Could you check a few things on this model? Use its own coordinates, in mm. A direction names the side the tool comes from. Round coordinates to 2 decimals unless told otherwise and drop trailing zeros. Write each loop counter-clockwise with the first axis right and the second up, starting at its lowest first coordinate (ties: lowest second). Pieces come first, ordered by that corner, then holes. Notation, with made-up numbers: M -17.75,-15 L 23.25,-15 A18 ccw 23.25,7 Z; hole C 22,48.5 d1. An arc over 180 degrees is marked long. One line per item, written item: value. Start each with the question number.
(1) Which directions (+Z, -Z, +X, -X, +Y, -Y) give clear straight access to the entire face, cutting with the end or side of a thin tool? Please do faces 4 (the face through (7, -66, 30)), 5 (the face through (1074.98, 1.66, 14.79)).
(2) Thinking about a two-plate mould opening in Y: for faces 1 (the face through (7, -66, 0)), 2 (the face through (1089.98, 1.99, 14.79)), 3 (the face through (-1049.99, -1.09, 14.79)), which applies, released by +Y, released by -Y, zero draft, split by the parting line, or undercut?
(3) I want a section at B-B on x = 436. Please give me the cut outline in (y, z).
(4) I want a section at C-C on z = 24. Please give me the cut outline in (x, y) (1 decimal), and give its area (3 significant figures).
(5) I want a section at A-A on y = 0. Please give me the cut outline in (x, z).
(6) I'm going to push flat-ended pins straight in: pin 1 Ø1 at (x, z) = (529, 23.5) entering from +Y; pin 2 Ø1.5 at (y, z) = (25, 26) entering from -X; pin 3 Ø4 at (y, z) = (44.5, 10.5) entering from -X. Where does each tip first touch, or does it pass through?
(7) If I drill on L1, parallel to X at y = 2.5, z = 17; L2, parallel to Y at x = 65.5, z = 23.75; L3, parallel to Y at x = -871, z = 24.5, over which ranges is the centre line in solid material (lowest first)?
Autodesk Inventor part; units mm, degrees
ref_plane "YZ Plane" through (0, 0, 0) normal (1, 0, 0) x (0, 1, 0)
ref_plane "XZ Plane" through (0, 0, 0) normal (0, 1, 0) x (-1, 0, 0)
ref_plane "XY Plane" through (0, 0, 0) normal (0, 0, 1) x (1, 0, 0)
sketch "Boceto1" plane through (0, 0, 0) normal (0, 0, 1) x (1, 0, 0)
  arc A0 (-1000.625, 49.9961) -> (-1000.625, -49.9961) centre (-1000, 0) ccw
  arc A1 (999.0625, -74.9941) -> (999.0625, 74.9941) centre (1000, 0) ccw
  line L0 (999.0625, 74.9941) -> (-1000.625, 49.9961)
  line L1 (-1000.625, -49.9961) -> (999.0625, -74.9941)
  line L2 (-1000.8125, 64.9949) -> (998.875, 89.993)
  arc A2 (998.875, -89.993) -> (998.875, 89.993) centre (1000, 0) ccw
  line L3 (998.875, -89.993) -> (-1000.8125, -64.9949)
  arc A3 (-1000.8125, 64.9949) -> (-1000.8125, -64.9949) centre (-1000, 0) ccw
  point P0 (0, 0)
  dimension "d0" = 2000
  dimension "d1" = 1000
  dimension "d2" = 100
  dimension "d3" = 150
  dimension "d4" = 15
extrude "Extrusión1" add sketch "Boceto1" along normal blind 30
properties part number "cadena"
Found:
1. face 4: +Z, +X, -X, +Y, -Y
1. face 5: +Z, -Z
2. face 1: zero draft
2. face 2: split by the parting line
2. face 3: undercut
3. outline: M -82.96,0 L -67.96,0 L -67.96,30 L -82.96,30 Z; M 67.96,0 L 82.96,0 L 82.96,30 L 67.96,30 Z
4. outline: M -1000.8,-65 L 998.9,-90 A90 ccw long 998.9,90 L -1000.8,65 A65 ccw Z; hole M -1000.6,-50 L 999.1,-75 A75 ccw long 999.1,75 L -1000.6,50 A50 ccw Z
4. area: 66,600 mm²
5. outline: M -1065,0 L -1050,0 L -1050,30 L -1065,30 Z; M 1075,0 L 1090,0 L 1090,30 L 1075,30 Z
6. pin 1: stops at y = 84.13
6. pin 2: stops at x = -1060.31
6. pin 3: stops at x = -1049.18
7. L1: x = -1064.95 to -1049.94, 1074.96 to 1089.97
7. L2: y = -78.32 to -63.32, 63.32 to 78.32
7. L3: y = -66.62 to -51.62, 51.62 to 66.62
